Model file for the job. Use its own axes, mm. A direction names the side the tool comes from. Give positions to 0.01 mm unless a question says otherwise; leave off trailing zeros. Loops run counter-clockwise (first coordinate to the right, second up) from the corner with the lowest first, then second, coordinate; pieces in that order, holes last. Notation, with made-up numbers: (-8.5, 35) - (9.5, 35) arc R26 ccw to (9.5, 59) - close; hole circle Ø4 at (-0.75, 72.5). An arc over 180 degrees is marked (long way). Answer as CSV lines item,"result". Start each with the question number.
Item 1: Drill centre lines: L1, parallel to X at y = 5, z = 4.5; L2, parallel to X at y = -5.5, z = 5; L3, parallel to Y at x = 4, z = 7. Where is each one in solid material? Low to high. Write a range as from..to.
Item 2: Saw through at B-B on z = 6. Give the cut face in (x, y).
Item 3: Pull direction Y, two halves, no side cores. Call faces 1 (the flat face through (3, 7.374, 4)), 2 (the cylindrical face through (2.46, 0.95, 4.09)), 3 (the flat face through (13, -8.126, 4)), 4 (the flat face through (0, 2, 3)): pulls with the +Y half, pulls with the -Y half, needs draft (parallel to the pull), parting line crosses it, or undercut.
Item 4: Saw through at D-D on y = -5.75. Give the cut face in (x, z).
Item 5: Pin check, flat tips, straight feed: pin 1 (2 mm diameter, centred on y = 2.5, z = 3.5, fed in from +X); pin 2 (1.5 mm diameter, centred on x = 11, z = 7, fed in from +Y); pin 3 (3 mm diameter, centred on y = -5, z = 5.5, fed in from -X). Stop position of each tip, or through.
Item 6: Tool access for faces 5 (the flat face through (5, 4, 4)), 6 (the flat face through (12.5, -5, 4)), 7 (the flat face through (5.4, -0.3, 9)): list every direction of +Z, -Z, +X, -X, +Y, -Y with a clear straight run to the whole face (end or side of a thin tool).
Item 7: Saw through at C-C on x = 2.5. Give the cut face in (y, z), plus the area to 3 significant figures.
Item 8: Saw through at A-A on y = 2.25. Give the cut face in (x, z).
from build123d import *

# Parameters (mm, degrees)
F1_DEPTH = 9
F2_R     = 1
F3_DEPTH = 25


with BuildPart() as f1:
    # F0 (on Top) → F1 (new body)
    with BuildSketch(Plane.XY):
        Polygon((5, 7.373742), (0, 7.373742), (0, -2.626258), (12.5, -2.626258), (12.5, -8.126258), (14.015152, -8.126258), (14.015152, -2.626258), (14.015152, 0), (5, 0), align=None)
    extrude(amount=F1_DEPTH)

    # F2 (on face) → F3 (cut)
    with BuildSketch(Plane(origin=(0, 0, 0), x_dir=(0, -1, 0), z_dir=(-1, 0, 0))):
        with Locations((-1.873742, 4.469738)):
            Circle(F2_R)
    extrude(amount=-F3_DEPTH, mode=Mode.SUBTRACT)


solid = f1.part
Responses:
1,L1,"0..5"
1,L2,"12.5..14.02"
1,L3,"-2.63..7.37"
2,outline,"(0, -2.63) - (12.5, -2.63) - (12.5, -8.13) - (14.02, -8.13) - (14.02, 0) - (5, 0) - (5, 7.37) - (0, 7.37) - close"
3,face 1,"pulls with the +Y half"
3,face 2,"undercut"
3,face 3,"pulls with the -Y half"
3,face 4,"needs draft"
4,outline,"(12.5, 0) - (14.02, 0) - (14.02, 9) - (12.5, 9) - close"
5,pin 1,"x = 5"
5,pin 2,"y = 0"
5,pin 3,"x = 12.5"
6,face 5,"+Z, -Z, +X, +Y"
6,face 6,"+Z, -Z, -X, -Y"
6,face 7,"+Z, +X, -X, +Y, -Y"
7,outline,"(-2.63, 0) - (7.37, 0) - (7.37, 9) - (-2.63, 9) - close; hole circle Ø2 at (1.87, 4.47)"
7,area,"86.9 mm2"
8,outline,"(0, 0) - (5, 0) - (5, 3.54) - (0, 3.54) - close; (0, 5.4) - (5, 5.4) - (5, 9) - (0, 9) - close"
